```python
from build123d import *

# Parameters (mm, degrees)
SKETCH1_R           = 3.96875
BOSS_EXTRUDE1_DEPTH = 6.35
BOSS_EXTRUDE2_DEPTH = 19.05
SKETCH4_R           = 3.96875
BOSS_EXTRUDE3_DEPTH = 6.35


with BuildPart() as part:
    # Sketch1 → Boss-Extrude1 (new body)
    with BuildSketch(Plane.XY):
        with BuildLine():
            Line((105.95, 8.85), (36.5125, 8.85))
            Line((36.5125, 8.85), (36.5125, 8.35))
            ThreePointArc((36.5125, 8.35), (35.926713562, 6.935786438), (34.5125, 6.35))
            Line((34.5125, 6.35), (-4.35, 6.35))
            ThreePointArc((-4.35, 6.35), (-5.764213562, 5.764213562), (-6.35, 4.35))
            Line((-6.35, 4.35), (-6.35, 0))
            ThreePointArc((-6.35, 0), (-4.490128061, -4.490128061), (0, -6.35))
            ThreePointArc((0, -6.35), (3.915636357, -4.999029097), (6.165159082, -1.520958084))
            ThreePointArc((6.165159082, -1.520958084), (6.873670176, -0.425502647), (8.10694147, 0))
            Line((8.10694147, 0), (93.49305853, 0))
            ThreePointArc((93.49305853, 0), (94.726329824, -0.425502647), (95.434840918, -1.520958084))
            ThreePointArc((95.434840918, -1.520958084), (97.684363643, -4.999029097), (101.6, -6.35))
            ThreePointArc((101.6, -6.35), (106.090128061, -4.490128061), (107.95, 0))
            Line((107.95, 0), (107.95, 6.85))
            ThreePointArc((107.95, 6.85), (107.364213562, 8.264213562), (105.95, 8.85))
        make_face()
        Circle(SKETCH1_R, mode=Mode.SUBTRACT)
        with Locations((101.6, 0)):
            Circle(SKETCH1_R, mode=Mode.SUBTRACT)
    extrude(amount=BOSS_EXTRUDE1_DEPTH)

    # Sketch3 → Boss-Extrude2 (add)
    with BuildSketch(Plane.XY.offset(6.35)):
        with BuildLine():
            Line((91.49305853, 6.35), (10.10694147, 6.35))
            ThreePointArc((10.10694147, 6.35), (8.692727908, 5.764213562), (8.10694147, 4.35))
            Line((8.10694147, 4.35), (8.10694147, 2))
            ThreePointArc((8.10694147, 2), (8.692727908, 0.585786438), (10.10694147, 0))
            Line((10.10694147, 0), (91.49305853, 0))
            ThreePointArc((91.49305853, 0), (92.907272092, 0.585786438), (93.49305853, 2))
            Line((93.49305853, 2), (93.49305853, 4.35))
            ThreePointArc((93.49305853, 4.35), (92.907272092, 5.764213562), (91.49305853, 6.35))
        make_face()
    extrude(amount=BOSS_EXTRUDE2_DEPTH)

    # Sketch4 → Boss-Extrude3 (add)
    with BuildSketch(Plane.XY.offset(25.4)):
        with BuildLine():
            Line((-4.35, 6.35), (34.5125, 6.35))
            ThreePointArc((34.5125, 6.35), (35.926713562, 6.935786438), (36.5125, 8.35))
            Line((36.5125, 8.35), (36.5125, 8.85))
            Line((36.5125, 8.85), (105.95, 8.85))
            ThreePointArc((105.95, 8.85), (107.364213562, 8.264213562), (107.95, 6.85))
            Line((107.95, 6.85), (107.95, 0))
            ThreePointArc((107.95, 0), (106.090128061, -4.490128061), (101.6, -6.35))
            ThreePointArc((101.6, -6.35), (97.684363643, -4.999029097), (95.434840918, -1.520958084))
            ThreePointArc((95.434840918, -1.520958084), (94.726329824, -0.425502647), (93.49305853, 0))
            Line((93.49305853, 0), (8.10694147, 0))
            ThreePointArc((8.10694147, 0), (6.873670176, -0.425502647), (6.165159082, -1.520958084))
            ThreePointArc((6.165159082, -1.520958084), (3.915636357, -4.999029097), (0, -6.35))
            ThreePointArc((0, -6.35), (-4.490128061, -4.490128061), (-6.35, 0))
            Line((-6.35, 0), (-6.35, 4.35))
            ThreePointArc((-6.35, 4.35), (-5.764213562, 5.764213562), (-4.35, 6.35))
        make_face()
        Circle(SKETCH4_R, mode=Mode.SUBTRACT)
        with Locations((101.6, 0)):
            Circle(SKETCH4_R, mode=Mode.SUBTRACT)
    extrude(amount=BOSS_EXTRUDE3_DEPTH)


solid = part.part
```
Source: CAD feature listing. Evaluate the final solid. Frame: model axes, mm. A direction names the side the tool comes from. Coordinates: 2 decimals unless noted, no trailing zeros. Loops run counter-clockwise (first coordinate to the right, second up) from the corner with the lowest first, then second, coordinate; pieces in that order, holes last. Notation, with made-up numbers: M 84.25,15 L 92.25,15 A24 ccw 92.25,39 Z; hole C 37,42 d8. An arc over 180 degrees is marked long. Put each result on its own line as item: value. Start each with the question number.
1) Contact query for flat-ended pins moving along their axis: pin 1 Ø2 at (x, z) = (71.5, 22) entering from -Y; pin 2 Ø1.9 at (y, z) = (3.5, 12.5) entering from -X; pin 3 Ø2.5 at (y, z) = (3, 19.5) entering from +X. Output: stop coordinate, or through.
2) Ray query, L1, parallel to Z at x = 3.5, y = 4.5; L2, parallel to Y at x = 0, z = 27.75; L3, parallel to Y at x = 55, z = 27.5. Return the intervals inside material, ascending. Write a range as from..to.
3) Cut plane C-C on x = 45. Return the cut outline in (y, z), then the cut area to 3 significant figures.
4) Cut plane D-D on z = 12.5. Return the cut outline in (x, y), then the cut area to 3 significant figures.
5) Reachability of faces 4 (the face through (6.888, -0.414, 28.531)), 5 (the face through (8.68, 0.6, 15.74)), 6 (the face through (92.92, 5.75, 15.74)), 7 (the face through (93.493, 3, 16)), 8 (the face through (8.107, 3, 16)) from +Z, -Z, +X, -X, +Y, -Y: full face, straight path, thin tool, end or side. Return the list, or none.
6) Cut plane A-A on x = 101.6. Return the cut outline in (y, z), then the cut area to 3 significant figures.
7) Cut plane B-B on z = 27.5. Return the cut outline in (x, y), then the cut area to 3 significant figures.
8) Pull-direction query (Z, two-part tool) for faces 1 (the face through (107.95, 3, 29)), 2 (the face through (50, 5, 0)), 3 (the face through (4, 2, 25.4)); classes: pulls with the +Z half, pulls with the -Z half, needs draft (parallel to the pull), parting line crosses it, or undercut.
The answers:
1. pin 1: stops at y = 0
1. pin 2: stops at x = 8.11
1. pin 3: stops at x = 93.49
2. L1: z = 0..6.35, 25.4..31.75
2. L2: y = -6.35..-3.97, 3.97..6.35
2. L3: y = 0..8.85
3. outline: M 0,0 L 8.85,0 L 8.85,6.35 L 6.35,6.35 L 6.35,25.4 L 8.85,25.4 L 8.85,31.75 L 0,31.75 Z
3. area: 233 mm²
4. outline: M 8.11,2 A2 ccw 10.11,0 L 91.49,0 A2 ccw 93.49,2 L 93.49,4.35 A2 ccw 91.49,6.35 L 10.11,6.35 A2 ccw 8.11,4.35 Z
4. area: 539 mm²
5. face 4: +Z, -Z, -Y
5. face 5: -X, -Y
5. face 6: +X, +Y
5. face 7: +X, +Y, -Y
5. face 8: -X, +Y, -Y
6. outline: M -6.35,0 L -3.97,0 L -3.97,6.35 L -6.35,6.35 Z; M -6.35,25.4 L -3.97,25.4 L -3.97,31.75 L -6.35,31.75 Z; M 3.97,0 L 8.85,0 L 8.85,6.35 L 3.97,6.35 Z; M 3.97,25.4 L 8.85,25.4 L 8.85,31.75 L 3.97,31.75 Z
6. area: 92.2 mm²
7. outline: M -6.35,0 A6.35 ccw 6.17,-1.52 A2 cw 8.11,0 L 93.49,0 A2 cw 95.43,-1.52 A6.35 ccw 107.95,0 L 107.95,6.85 A2 ccw 105.95,8.85 L 36.51,8.85 L 36.51,8.35 A2 cw 34.51,6.35 L -4.35,6.35 A2 ccw -6.35,4.35 Z; hole C 0,0 d7.94; hole C 101.6,0 d7.94
7. area: 932 mm²
8. face 1: needs draft
8. face 2: pulls with the -Z half
8. face 3: undercut
